Autodesk Inventor part; units mm, degrees
ref_plane "YZ Plane" through (0, 0, 0) normal (1, 0, 0) x (0, 1, 0)
ref_plane "XZ Plane" through (0, 0, 0) normal (0, 1, 0) x (-1, 0, 0)
ref_plane "XY Plane" through (0, 0, 0) normal (0, 0, 1) x (1, 0, 0)
sketch "スケッチ1" plane through (0, 0, 0) normal (0, 0, 1) x (1, 0, 0)
  line L0 (-47.5, 5.75) -> (47.5, 5.75)
  line L1 (47.5, 5.75) -> (47.5, -5.75)
  line L2 (47.5, -5.75) -> (-47.5, -5.75)
  line L3 (-47.5, -5.75) -> (-47.5, 5.75)
  line L4 (-47.5, 5.75) -> (47.5, -5.75) construction
  line L5 (47.5, 5.75) -> (-47.5, -5.75) construction
  point P0 (0, 0)
  dimension "d0" = 11.5
  dimension "d1" = 95
extrude "押し出し1" add sketch "スケッチ1" along normal blind 1.5
sketch "スケッチ2" plane through (0, 0, 1.5) normal (0, 0, 1) x (1, 0, 0)
  line L0 (-42.5, 2.3) -> (42.5, 2.3)
  line L1 (42.5, 2.3) -> (42.5, -0.8)
  line L2 (42.5, -0.8) -> (-42.5, -0.8)
  line L3 (-42.5, -0.8) -> (-42.5, 2.3)
  line L4 (-47.5, -5.75) -> (47.5, -5.75)
  line L5 (47.5, -5.75) -> (47.5, 5.75)
  point P0 (0, 0)
  dimension "d8" = 3.1
  dimension "d9" = 85
  dimension "d10" = 4.95
  dimension "d11" = 5
extrude "押し出し2" cut sketch "スケッチ2" against normal blind 1.5
sketch "スケッチ5" plane through (-47.5, 5.75, 0) normal (0, 1, 0) x (1, 0, 0)
  line L0 (0, 0) -> (95, 0)
  line L1 (95, 0) -> (95, -1.5)
  line L2 (95, -1.5) -> (0, -1.5)
  line L3 (0, -1.5) -> (0, 0)
  point P0 (47.5, 0)
extrude "押し出し4" add sketch "スケッチ5" along normal blind 20
sketch "スケッチ6" plane through (0, 0, 1.5) normal (0, 0, 1) x (1, 0, 0)
  line L0 (-47.5, 25.75) -> (47.5, 25.75)
  line L1 (-47.5, -5.75) -> (-47.5, 25.75)
  point P0 (0, 0)
  point P1 (30.5, 22.25)
  point P2 (-30.5, 22.25)
  point P3 (-30.5, 14.25)
  point P4 (30.5, 14.25)
  dimension "d32" = 3.5
  dimension "d33" = 8
  dimension "d34" = 61
  dimension "d35" = 17
hole "穴2" at (30.5, 22.25, 1.5) at (-30.5, 22.25, 1.5) at (-30.5, 14.25, 1.5) at (30.5, 14.25, 1.5) direction (0, 0, -1) diameter 3.1 end through all
equation "\"d41\" = Thickness"
equation "\"BendRadius\" = Thickness"
equation "\"BendReliefWidth\" = Thickness"
equation "\"BendReliefDepth\" = 0.5 * Thickness"
equation "\"CornerReliefSize\" = 4 * Thickness"
equation "\"MinimumRemnant\" = 2 * Thickness"
equation "\"TransitionRadius\" = BendRadius"
equation "\"JacobiRadiusSize\" = BendRadius"
equation "\"GapSize\" = Thickness"
properties part number "Fork 2 ver2c" material "アルミニウム 5052 H32"
Here's how the part is built. I have some questions about the finished solid (model axes, mm). Round coordinates to 2 decimals unless told otherwise and drop trailing zeros. Loops run counter-clockwise (first coordinate to the right, second up) from the corner with the lowest first, then second, coordinate; pieces in that order, holes last. Notation, with made-up numbers: (78.5, 12.25) -> (92.5, 12.25) arc R17 ccw to (92.5, 25.25) -> close; hole circle Ø6 at (30, -25). An arc over 180 degrees is marked (long way). Answer as CSV lines item,"result".
1. Thinking about a two-plate mould opening in Y: for faces 1 (the face through (-32.037, 14.452, 0.74)), 2 (the face through (29.45, 15.39, 0.74)), 3 (the face through (-1, 10, 0)), which applies, released by +Y, released by -Y, zero draft, split by the parting line, or undercut?
Final values:
face 1,"undercut"
face 2,"undercut"
face 3,"zero draft"
2. If we section it at B-B on z = 1.1: Please give me the cut outline in (x, y), plus the area to 3 significant figures.
Final values:
outline,"(-47.5, -5.75) -> (47.5, -5.75) -> (47.5, 25.75) -> (-47.5, 25.75) -> close; hole (-42.5, -0.8) -> (42.5, -0.8) -> (42.5, 2.3) -> (-42.5, 2.3) -> close; hole circle Ø3.1 at (-30.5, 14.25); hole circle Ø3.1 at (-30.5, 22.25); hole circle Ø3.1 at (30.5, 14.25); hole circle Ø3.1 at (30.5, 22.25)"
area,"2,700 mm^2"
3. If we section it at A-A on y = 1: Please give me the cut outline in (x, z).
Final values:
outline,"(-47.5, 0) -> (-42.5, 0) -> (-42.5, 1.5) -> (-47.5, 1.5) -> close; (42.5, 0) -> (47.5, 0) -> (47.5, 1.5) -> (42.5, 1.5) -> close"
4. If we section it at D-D on y = 14.25: Please give me the cut outline in (x, z), plus the area to 3 significant figures.
Final values:
outline,"(-47.5, 0) -> (-32.05, 0) -> (-32.05, 1.5) -> (-47.5, 1.5) -> close; (-28.95, 0) -> (28.95, 0) -> (28.95, 1.5) -> (-28.95, 1.5) -> close; (32.05, 0) -> (47.5, 0) -> (47.5, 1.5) -> (32.05, 1.5) -> close"
area,"133 mm^2"
5. If we section it at C-C on x = -34: Please give me the cut outline in (y, z).
Final values:
outline,"(-5.75, 0) -> (-0.8, 0) -> (-0.8, 1.5) -> (-5.75, 1.5) -> close; (2.3, 0) -> (25.75, 0) -> (25.75, 1.5) -> (2.3, 1.5) -> close"
6. If I drill on L1, parallel to Y at x = -30.5, z = 0.5; L2, parallel to X at y = 14.25, z = 0.85; L3, parallel to Y at x = -40, z = 0.35, over which ranges is the centre line in solid material (lowest first)?
Final values:
L1,"y = -5.75 to -0.8, 2.3 to 12.7, 15.8 to 20.7, 23.8 to 25.75"
L2,"x = -47.5 to -32.05, -28.95 to 28.95, 32.05 to 47.5"
L3,"y = -5.75 to -0.8, 2.3 to 25.75"
7. For pin 1 (3 mm diameter, centred on x = 30.5, y = 22.25, fed in from +Z), with a flat end and sliding along its axis, tell me the tip position at first contact or that it passes through.
Final values:
pin 1,"passes through"
